For this review, take the finished solid that the model builds, in its own axes (mm). Give positions to 0.01 mm unless a question says otherwise; leave off trailing zeros. Loops run counter-clockwise (first coordinate to the right, second up) from the corner with the lowest first, then second, coordinate; pieces in that order, holes last.
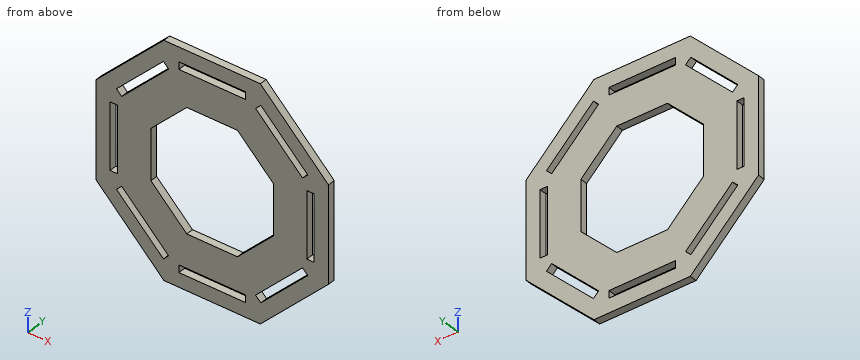
Autodesk Inventor part; units mm, degrees
ref_plane "YZ Plane" through (0, 0, 0) normal (1, 0, 0) x (0, 1, 0)
ref_plane "XZ Plane" through (0, 0, 0) normal (0, 1, 0) x (-1, 0, 0)
ref_plane "XY Plane" through (0, 0, 0) normal (0, 0, 1) x (1, 0, 0)
sketch "Sketch1" plane through (0, 0, 0) normal (0, 1, 0) x (-1, 0, 0)
  line L0 (-14.2875, -40.7478) -> (14.2875, -40.7478)
  line L1 (14.2875, -40.7478) -> (14.2875, -43.9228)
  line L2 (14.2875, -43.9228) -> (-14.2875, -43.9228)
  line L3 (-14.2875, -43.9228) -> (-14.2875, -40.7478)
  line L4 (18.7102, -38.9158) -> (38.9158, -18.7102)
  line L5 (38.9158, -18.7102) -> (41.1609, -20.9553)
  line L6 (41.1609, -20.9553) -> (20.9553, -41.1609)
  line L7 (20.9553, -41.1609) -> (18.7102, -38.9158)
  line L8 (40.7478, -14.2875) -> (40.7478, 14.2875)
  line L9 (40.7478, 14.2875) -> (43.9228, 14.2875)
  line L10 (43.9228, 14.2875) -> (43.9228, -14.2875)
  line L11 (43.9228, -14.2875) -> (40.7478, -14.2875)
  line L12 (38.9158, 18.7102) -> (18.7102, 38.9158)
  line L13 (18.7102, 38.9158) -> (20.9553, 41.1609)
  line L14 (20.9553, 41.1609) -> (41.1609, 20.9553)
  line L15 (41.1609, 20.9553) -> (38.9158, 18.7102)
  line L16 (14.2875, 40.7478) -> (-14.2875, 40.7478)
  line L17 (-14.2875, 40.7478) -> (-14.2875, 43.9228)
  line L18 (-14.2875, 43.9228) -> (14.2875, 43.9228)
  line L19 (14.2875, 43.9228) -> (14.2875, 40.7478)
  line L20 (-18.7102, 38.9158) -> (-38.9158, 18.7102)
  line L21 (-38.9158, 18.7102) -> (-41.1609, 20.9553)
  line L22 (-41.1609, 20.9553) -> (-20.9553, 41.1609)
  line L23 (-20.9553, 41.1609) -> (-18.7102, 38.9158)
  line L24 (-40.7478, 14.2875) -> (-40.7478, -14.2875)
  line L25 (-40.7478, -14.2875) -> (-43.9228, -14.2875)
  line L26 (-43.9228, -14.2875) -> (-43.9228, 14.2875)
  line L27 (-43.9228, 14.2875) -> (-40.7478, 14.2875)
  line L28 (-38.9158, -18.7102) -> (-18.7102, -38.9158)
  line L29 (-18.7102, -38.9158) -> (-20.9553, -41.1609)
  line L30 (-20.9553, -41.1609) -> (-41.1609, -20.9553)
  line L31 (-41.1609, -20.9553) -> (-38.9158, -18.7102)
  line L32 (50.0728, -20.7409) -> (20.7409, -50.0728)
  line L33 (20.7409, -50.0728) -> (-20.7409, -50.0728)
  line L34 (-20.7409, -50.0728) -> (-50.0728, -20.7409)
  line L35 (-50.0728, -20.7409) -> (-50.0728, 20.7409)
  line L36 (-50.0728, 20.7409) -> (-20.7409, 50.0728)
  line L37 (-20.7409, 50.0728) -> (20.7409, 50.0728)
  line L38 (20.7409, 50.0728) -> (50.0728, 20.7409)
  line L39 (50.0728, 20.7409) -> (50.0728, -20.7409)
  line L40 (26.3506, -10.9148) -> (10.9148, -26.3506)
  line L41 (10.9148, -26.3506) -> (-10.9148, -26.3506)
  line L42 (-10.9148, -26.3506) -> (-26.3506, -10.9148)
  line L43 (-26.3506, -10.9148) -> (-26.3506, 10.9148)
  line L44 (-26.3506, 10.9148) -> (-10.9148, 26.3506)
  line L45 (-10.9148, 26.3506) -> (10.9148, 26.3506)
  line L46 (10.9148, 26.3506) -> (26.3506, 10.9148)
  line L47 (26.3506, 10.9148) -> (26.3506, -10.9148)
  point P0 (0, 0)
  point P1 (0, 0)
  point P2 (0, 0)
  point P3 (0, 0)
  dimension "d0" = 28.575
  dimension "d1" = 3.175
  dimension "d2" = 43.18
  dimension "d3" = 43.18
  dimension "d6" = 360
extrude "Extrusion1" add sketch "Sketch1" along normal blind 3.175
properties part number "octoBotoStemRingLarger01"
Q1. Consider section D-D on x = -29. Give the boundary of the cut face in (y, z) (3 decimals).
Answers:
outline: (0, -41.814) - (3.175, -41.814) - (3.175, -33.116) - (0, -33.116) - close; (0, -28.626) - (3.175, -28.626) - (3.175, 28.626) - (0, 28.626) - close; (0, 33.116) - (3.175, 33.116) - (3.175, 41.814) - (0, 41.814) - close
Q2. Consider section A-A on z = -7.5. Give the boundary of the cut face in (x, y) (3 decimals), plus the area to 3 significant figures.
Answers:
outline: (-50.073, 0) - (-43.923, 0) - (-43.923, 3.175) - (-50.073, 3.175) - close; (-40.748, 0) - (-26.351, 0) - (-26.351, 3.175) - (-40.748, 3.175) - close; (26.351, 0) - (40.748, 0) - (40.748, 3.175) - (26.351, 3.175) - close; (43.923, 0) - (50.073, 0) - (50.073, 3.175) - (43.923, 3.175) - close
area: 130 mm2
Q3. For probe 1 along X at (y, z) = (0.5, -10); probe 2 along Z at (x, y) = (27.5, 1.05); probe 3 along X at (y, z) = (1.6, 39), list the stretches that pass through material, from the lowest coordinate up.
Answers:
probe 1: x = -50.07 to -43.92, -40.75 to -26.35, 26.35 to 40.75, 43.92 to 50.07
probe 2: z = -43.31 to -34.62, -30.13 to 30.13, 34.62 to 43.31
probe 3: x = -31.81 to -23.12, -18.79 to 18.79, 23.12 to 31.81
Q4. Consider section B-B on x = 1.5. Give the boundary of the cut face in (y, z) (3 decimals).
Answers:
outline: (0, -50.073) - (3.175, -50.073) - (3.175, -43.923) - (0, -43.923) - close; (0, -40.748) - (3.175, -40.748) - (3.175, -26.351) - (0, -26.351) - close; (0, 26.351) - (3.175, 26.351) - (3.175, 40.748) - (0, 40.748) - close; (0, 43.923) - (3.175, 43.923) - (3.175, 50.073) - (0, 50.073) - close
Q5. For pin 1 Ø1 at (x, y) = (43, 1.5) entering from +Z; pin 2 Ø1 at (x, y) = (-42.5, 2) entering from -Z; pin 3 Ø4 at (x, z) = (-36, 6) entering from -Y, all flat-tipped, find the tip position at first contact; note any pin that passes through.
Answers:
pin 1: stops at z = 28.31
pin 2: stops at z = -28.81
pin 3: stops at y = 0
Q6. Consider section C-C on z = 36. Give the boundary of the cut face in (x, y) (3 decimals), plus the area to 3 significant figures.
Answers:
outline: (-34.814, 0) - (-26.116, 0) - (-26.116, 3.175) - (-34.814, 3.175) - close; (-21.626, 0) - (21.626, 0) - (21.626, 3.175) - (-21.626, 3.175) - close; (26.116, 0) - (34.814, 0) - (34.814, 3.175) - (26.116, 3.175) - close
area: 193 mm2
